```python
from build123d import *

# Parameters (mm, degrees)
VARIOUS_MOUNTING_POINTS_DEPTH      = 302.472328172
VARIOUS_MOUNTING_POINTS_DEPTH_BACK = 302.472328172
SKETCH4_R                          = 5
SKETCH5_W                          = 142.042704148
SKETCH5_H                          = 92.874075788
CUT_EXTRUDE1_DEPTH                 = 422.289527912


with BuildPart() as part:
    # Sweep1: sweep along a path in Sketch3
    with BuildLine(Plane(origin=(0, 0, 0), x_dir=(0, 0, -1), z_dir=(1, 0, 0))) as sweep1_path:
        ThreePointArc((-240, -6), (30, 0.074962051), (300, -6))
    # Sketch1 → Sweep1 (sweep)
    with BuildSketch(Plane.XY):
        with BuildLine():
            Line((-17, 0), (17, 0))
            ThreePointArc((17, 0), (19.121320344, 0.878679656), (20, 3))
            Line((20, 3), (20, 10))
            Line((20, 10), (22, 10))
            Line((22, 10), (22, -2))
            Line((22, -2), (-22, -2))
            Line((-22, -2), (-22, 10))
            Line((-22, 10), (-20, 10))
            Line((-20, 10), (-20, 3))
            ThreePointArc((-20, 3), (-19.121320344, 0.878679656), (-17, 0))
        make_face()
    sweep(path=sweep1_path.line)

    # Sketch4 → Various mounting points (cut, two sides: drawn at the far end of the back side and taken through both)
    with BuildSketch(Plane(origin=(0, 0, 0), x_dir=(1, 0, 0), z_dir=(0, 1, 0)).offset(-VARIOUS_MOUNTING_POINTS_DEPTH_BACK)):
        with Locations(Location((0, 197.900062461, 0), (0, 0, 270))):
            Circle(SKETCH4_R)
        with Locations(Location((0, -223.099937539, 0), (0, 0, 270))):
            Circle(SKETCH4_R)
        with BuildLine():
            Line((-5, 256.900062461), (-5, 276.900062461))
            ThreePointArc((-5, 276.900062461), (0, 281.900062461), (5, 276.900062461))
            Line((5, 276.900062461), (5, 256.900062461))
            ThreePointArc((5, 256.900062461), (0, 251.900062461), (-5, 256.900062461))
        make_face()
        with BuildLine():
            Line((-5, 87.900062461), (-5, 107.900062461))
            ThreePointArc((-5, 107.900062461), (0, 112.900062461), (5, 107.900062461))
            Line((5, 107.900062461), (5, 87.900062461))
            ThreePointArc((5, 87.900062461), (0, 82.900062461), (-5, 87.900062461))
        make_face()
        with BuildLine():
            Line((-5, 7.900062461), (-5, 27.900062461))
            ThreePointArc((-5, 27.900062461), (0, 32.900062461), (5, 27.900062461))
            Line((5, 27.900062461), (5, 7.900062461))
            ThreePointArc((5, 7.900062461), (0, 2.900062461), (-5, 7.900062461))
        make_face()
        with BuildLine():
            Line((-5, -72.099937539), (-5, -52.099937539))
            ThreePointArc((-5, -52.099937539), (0, -47.099937539), (5, -52.099937539))
            Line((5, -52.099937539), (5, -72.099937539))
            ThreePointArc((5, -72.099937539), (0, -77.099937539), (-5, -72.099937539))
        make_face()
        with BuildLine():
            Line((-5, -152.099937539), (-5, -132.099937539))
            ThreePointArc((-5, -132.099937539), (0, -127.099937539), (5, -132.099937539))
            Line((5, -132.099937539), (5, -152.099937539))
            ThreePointArc((5, -152.099937539), (0, -157.099937539), (-5, -152.099937539))
        make_face()
    extrude(amount=VARIOUS_MOUNTING_POINTS_DEPTH + VARIOUS_MOUNTING_POINTS_DEPTH_BACK, mode=Mode.SUBTRACT)

    # Sketch5 → Cut-Extrude1 (cut, through all)
    with BuildSketch(Plane(origin=(0, -4.799999233, 119.951980823), x_dir=(1, 0, 0), z_dir=(0, -0.039984006397440985, 0.9992003198720513))):
        with Locations((-10.646198733, -6.327716956)):
            Rectangle(SKETCH5_W, SKETCH5_H)
    extrude(amount=-CUT_EXTRUDE1_DEPTH, mode=Mode.SUBTRACT)


solid = part.part
```
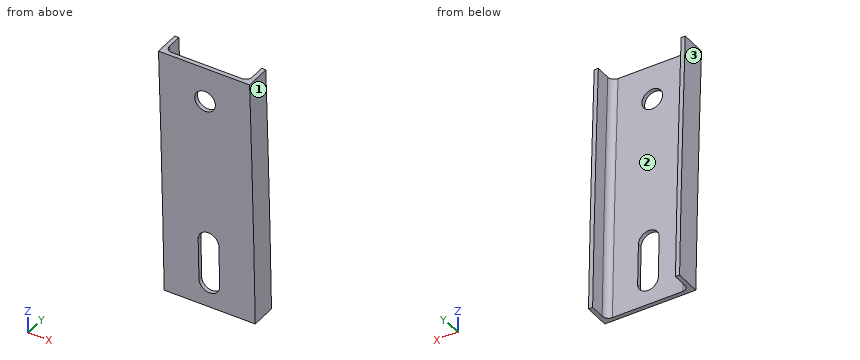
For this review, take the finished solid that the model builds, in its own axes (mm). Face numbers are marked on the shaded views. Coordinates: 2 decimals unless noted, no trailing zeros. Loops run counter-clockwise (first coordinate to the right, second up) from the corner with the lowest first, then second, coordinate; pieces in that order, holes last. Notation, with made-up numbers: (-10, 60.25) - (11, 60.25) arc R24 ccw to (11, 72.25) - close; hole circle Ø7 at (-26.5, -8.75). An arc over 180 degrees is marked (long way). Use one line per item in the form item = value. Start each with the question number.
1) For pin 1 (12 mm diameter, centred on x = 10, z = 184, fed in from -Y); pin 2 (10 mm diameter, centred on x = -3.5, z = 142, fed in from -Y); pin 3 (8 mm diameter, centred on x = 0, z = 223.1, fed in from +Y); pin 4 (2 mm diameter, centred on x = 12.5, z = 138.5, fed in from +Y), all flat-tipped, find the tip position at first contact; note any pin that passes through.
2) To check wall thickness, follow probe 1 along X at (y, z) = (3.75, 222); probe 2 along X at (y, z) = (-1.25, 143); probe 3 along Y at (x, z) = (18, 153). State the ranges of each line that lie inside material, in increasing order. Write a range as from..to.
3) Take a section at B-B (x = -9.5). State the section outline as (y, z) points.
4) Take a section at A-A (x = 0). State the section outline as (y, z) points.
5) Draft analysis for pull direction X (two halves, no side actions). For the marked faces 1, 2 and 3, state which applies: released by +X, released by -X, zero draft, split by the parting line, or undercut.
From the geometry:
q1.pin_1 = -5.96
q1.pin_2 = -4.53
q1.pin_3 = through
q1.pin_4 = -2.26
q2.probe_1 = -22..-20, 20..22
q2.probe_2 = -22..-19.38, 19.38..22
q2.probe_3 = -4.72..-2.54
q3.outline = (-8, 239.92) arc R6001.07 cw to (-3.8, 119.99) - (-1.8, 120.07) arc R6003.07 ccw to (-6, 240) - close
q4.outline = (-8, 239.92) arc R6001.07 cw to (-7.48, 228.1) - (-5.48, 228.1) arc R6003.07 ccw to (-6, 240) - close; (-7.06, 218.1) arc R6001.07 cw to (-4.84, 157.1) - (-2.84, 157.1) arc R6003.07 ccw to (-5.05, 218.1) - close; (-3.98, 127.1) arc R6001.07 cw to (-3.8, 119.99) - (-1.8, 120.07) arc R6003.07 ccw to (-1.98, 127.1) - close
q5.face_1 = released by +X
q5.face_2 = undercut
q5.face_3 = released by -X
